```python
from build123d import *

# Parameters (mm, degrees)
PAD_DEPTH       = 10
SKETCH001_W     = 9
SKETCH001_H     = 3.2
SKETCH001_W_2   = 15
SKETCH001_H_2   = 5.5
SKETCH001_H_3   = 5
SKETCH001_W_3   = 16.5
SKETCH001_H_4   = 14
SKETCH001_W_4   = 16
SKETCH001_H_5   = 16
SKETCH001_W_5   = 17
POCKET_DEPTH    = 2
SKETCH002_R     = 12
POCKET001_DEPTH = 8
SKETCH003_W     = 41
SKETCH003_H     = 19
POCKET002_DEPTH = 8
SKETCH004_W     = 35
SKETCH004_H     = 12.5
POCKET003_DEPTH = 8
SKETCH005_W     = 41
SKETCH005_H     = 21
POCKET004_DEPTH = 8
SKETCH006_W     = 14
SKETCH006_H     = 12
POCKET005_DEPTH = 8
SKETCH007_W     = 13
SKETCH007_H     = 8
POCKET006_DEPTH = 8
SKETCH008_W     = 27
SKETCH008_H     = 10
POCKET007_DEPTH = 8
SKETCH009_W     = 23
SKETCH009_H     = 23
POCKET008_DEPTH = 8


with BuildPart() as part:
    # Sketch → Pad (new body)
    with BuildSketch(Plane.XY):
        Polygon((126.692246, 7.136342), (-0.047754, 7.136342), (-49.921126, -33.859272), (-50.819163, -43.341843), (1.360604, -57.146646), (104.980095, -56.822042), (126.692246, -27.893658), align=None)
    extrude(amount=PAD_DEPTH)

    # Sketch001 (on Face9 of Pad) → Pocket (cut)
    with BuildSketch(Plane.XY.offset(10)):
        with Locations((4.5, -14.55)):
            Rectangle(SKETCH001_W, SKETCH001_H)
        with Locations((4.5, -27.55)):
            Rectangle(SKETCH001_W, SKETCH001_H)
        with Locations((4.5, -40.55)):
            Rectangle(SKETCH001_W, SKETCH001_H)
        with Locations((67.5, -26.5)):
            Rectangle(SKETCH001_W_2, SKETCH001_H_2)
        with Locations((67.5, -7.5)):
            Rectangle(SKETCH001_W, SKETCH001_H_3)
        with Locations((101.5, -26.5)):
            Rectangle(SKETCH001_W_3, SKETCH001_H_4)
        with Locations((32, -13)):
            Rectangle(SKETCH001_W_4, SKETCH001_H_5)
        with Locations((32, -40)):
            Rectangle(SKETCH001_W_4, SKETCH001_H_5)
        with Locations((67.5, -45.25)):
            Rectangle(SKETCH001_W_5, SKETCH001_H_2)
    extrude(amount=-POCKET_DEPTH, mode=Mode.SUBTRACT)

    # Sketch002 (on Face4 of Pocket) → Pocket001 (cut)
    with BuildSketch(Plane(origin=(0, 0, 0), x_dir=(1, 0, 0), z_dir=(0, 0, -1))):
        with Locations((32, 39.982296)):
            Circle(SKETCH002_R)
        with Locations((32, 12.989247)):
            Circle(SKETCH002_R)
    extrude(amount=-POCKET001_DEPTH, mode=Mode.SUBTRACT)

    # Sketch003 (on Face4 of Pocket001) → Pocket002 (cut)
    with BuildSketch(Plane(origin=(0, 0, 0), x_dir=(1, 0, 0), z_dir=(0, 0, -1))):
        with Locations((67.481461, 7.5)):
            Rectangle(SKETCH003_W, SKETCH003_H)
    extrude(amount=-POCKET002_DEPTH, mode=Mode.SUBTRACT)

    # Sketch004 (on Face4 of Pocket002) → Pocket003 (cut)
    with BuildSketch(Plane(origin=(0, 0, 0), x_dir=(1, 0, 0), z_dir=(0, 0, -1))):
        with Locations((67.513935, 45.25)):
            Rectangle(SKETCH004_W, SKETCH004_H)
    extrude(amount=-POCKET003_DEPTH, mode=Mode.SUBTRACT)

    # Sketch005 (on Face4 of Pocket003) → Pocket004 (cut)
    with BuildSketch(Plane(origin=(0, 0, 0), x_dir=(1, 0, 0), z_dir=(0, 0, -1))):
        with Locations((67.69477, 26.497755)):
            Rectangle(SKETCH005_W, SKETCH005_H)
    extrude(amount=-POCKET004_DEPTH, mode=Mode.SUBTRACT)

    # Sketch006 (on Face4 of Pocket004) → Pocket005 (cut)
    with BuildSketch(Plane(origin=(0, 0, 0), x_dir=(1, 0, 0), z_dir=(0, 0, -1))):
        with Locations((4.509145, 40.540194)):
            Rectangle(SKETCH006_W, SKETCH006_H)
    extrude(amount=-POCKET005_DEPTH, mode=Mode.SUBTRACT)

    # Sketch007 (on Face4 of Pocket005) → Pocket006 (cut)
    with BuildSketch(Plane(origin=(0, 0, 0), x_dir=(1, 0, 0), z_dir=(0, 0, -1))):
        with Locations((4.5, 27.545833)):
            Rectangle(SKETCH007_W, SKETCH007_H)
    extrude(amount=-POCKET006_DEPTH, mode=Mode.SUBTRACT)

    # Sketch008 (on Face4 of Pocket006) → Pocket007 (cut)
    with BuildSketch(Plane(origin=(0, 0, 0), x_dir=(1, 0, 0), z_dir=(0, 0, -1))):
        with Locations((4.5, 14.554985)):
            Rectangle(SKETCH008_W, SKETCH008_H)
    extrude(amount=-POCKET007_DEPTH, mode=Mode.SUBTRACT)

    # Sketch009 (on Face4 of Pocket007) → Pocket008 (cut)
    with BuildSketch(Plane(origin=(0, 0, 0), x_dir=(1, 0, 0), z_dir=(0, 0, -1))):
        with Locations((101.5, 25)):
            Rectangle(SKETCH009_W, SKETCH009_H)
    extrude(amount=-POCKET008_DEPTH, mode=Mode.SUBTRACT)


solid = part.part
```
The listing builds one solid part. Answer for the finished solid, in the listing's coordinates (mm). A direction names the side the tool comes from. Coordinates: 2 decimals unless noted, no trailing zeros. Loops run counter-clockwise (first coordinate to the right, second up) from the corner with the lowest first, then second, coordinate; pieces in that order, holes last. Notation, with made-up numbers: (71.25, -32) - (83.25, -32) arc R11 ccw to (83.25, -12) - close; hole circle Ø1 at (-29, 70.25). An arc over 180 degrees is marked (long way). Use a Markdown table: item, result. Add a question column.
1) The part is cut by section B-B, the plane x = 101.5. Give the vertices of the cut face in (y, z), and give its area (3 significant figures).
2) The mould has two halves that part along X. Classify faces 1 (the flat face through (115.684, -42.56, 4.93)), 2 (the flat face through (37, -25, 10)), 3 (the flat face through (23, -41, 8)): released by +X, released by -X, zero draft, split by the parting line, or undercut.
3) The part is cut by section A-A, the plane x = 32. Give the vertices of the cut face in (y, z), and give its area (3 significant figures).
4) For faces 4 (the flat face through (67, -36.998, 4)), 5 (the flat face through (37, -25, 0)), determine the directions among +Z, -Z, +X, -X, +Y, -Y from which every point of the face is accessible in a straight line to the end or side of a thin tool.
5) The part is cut by section D-D, the plane z = 2.5. State how many separate pieces and enclosed holes the cut face has, and give its area (3 significant figures).
6) The part is cut by section C-C, the plane x = 80.5. Give the vertices of the cut face in (y, z), and give its area (3 significant figures).
7) Find the intervals of material crossed by line 1 (Y direction, x = 13, z = 1.75); line 2 (X direction, y = -15, z = 4.75); line 3 (Y direction, x = 32, z = 2.25), in increasing order.
8) Given pin 1 (4 mm diameter, centred on y = -16.5, z = 1, fed in from -X); pin 2 (2 mm diameter, centred on x = 6.5, z = 8.5, fed in from -Y); pin 3 (1.6 mm diameter, centred on y = -17, z = 9, fed in from -X), each flat-ended and moving along its own axis, determine where each tip first touches the part or whether it passes through.
Here are the results:
| question | item | result |
|---|---|---|
| 1 | outline | (-56.83, 0) - (-36.5, 0) - (-36.5, 8) - (-33.5, 8) - (-33.5, 10) - (-56.83, 10) - close; (-19.5, 8) - (-13.5, 8) - (-13.5, 0) - (7.14, 0) - (7.14, 10) - (-19.5, 10) - close |
| 1 | area | 428 mm^2 |
| 2 | face 1 | released by +X |
| 2 | face 2 | zero draft |
| 2 | face 3 | undercut |
| 3 | outline | (-57.05, 0) - (-51.98, 0) - (-51.98, 8) - (-48, 8) - (-48, 10) - (-57.05, 10) - close; (-32, 8) - (-27.98, 8) - (-27.98, 0) - (-24.99, 0) - (-24.99, 8) - (-21, 8) - (-21, 10) - (-32, 10) - close; (-5, 8) - (-0.99, 8) - (-0.99, 0) - (7.14, 0) - (7.14, 10) - (-5, 10) - close |
| 3 | area | 194 mm^2 |
| 4 | face 4 | -Z |
| 4 | face 5 | -Z, +X, -X, +Y, -Y |
| 5 | separate pieces | 1 |
| 5 | enclosed holes | 8 |
| 5 | area | 5,640 mm^2 |
| 6 | outline | (-56.9, 0) - (-51.5, 0) - (-51.5, 8) - (-39, 8) - (-39, 0) - (-37, 0) - (-37, 8) - (2, 8) - (2, 0) - (7.14, 0) - (7.14, 10) - (-56.9, 10) - close |
| 6 | area | 228 mm^2 |
| 7 | line 1 | y = -57.11 to -19.55, -9.55 to 7.14 |
| 7 | line 2 | x = -26.98 to -9, 18 to 20.17, 43.83 to 46.98, 87.98 to 90, 113 to 126.69 |
| 7 | line 3 | y = -57.05 to -51.98, -27.98 to -24.99, -0.99 to 7.14 |
| 8 | pin 1 | stops at x = -31.24 |
| 8 | pin 2 | stops at y = -57.13 |
| 8 | pin 3 | stops at x = -30.38 |
